Check sheet for the drawn part. Datum: minimum x, y, z corner. Units: mm. Coordinates: 2 decimals unless noted, no trailing zeros. Order: outer loops, then holes, each group sorted by start corner. A loop starts at its lowest first (then second) coordinate and runs counter-clockwise, first axis right, second up.
Q1. Cross-section at B-B, the plane x = 143. Record the boundary of the cut face in (y, z) (1 decimal), and give its area (3 significant figures).
Q2. Cross-section at A-A, the plane y = 4. Count the separate pieces of the cut face and the enclosed holes in it, and give its area (3 significant figures).
Q3. Depth check by flat-ended pin: P1, Ø3, axis at x = 66.5, y = 3, coming from the -Z side; P2, Ø3, axis at x = 112.5, y = 2.5, coming from the -Z side. Enter the tip coordinate at first touch or a pass-through.
Q4. Cross-section at C-C, the plane z = 89. Record the boundary of the cut face in (x, y) (1 decimal), and give its area (3 significant figures).
Q5. Thickness scan on line 1 (Z direction, x = 83.5, y = 4.35); line 2 (Z direction, x = 116.5, y = 4.7) (1 decimal); line 3 (X direction, y = 4.35, z = 144.5) (1 decimal). Record the ranges inside material, lowest first.
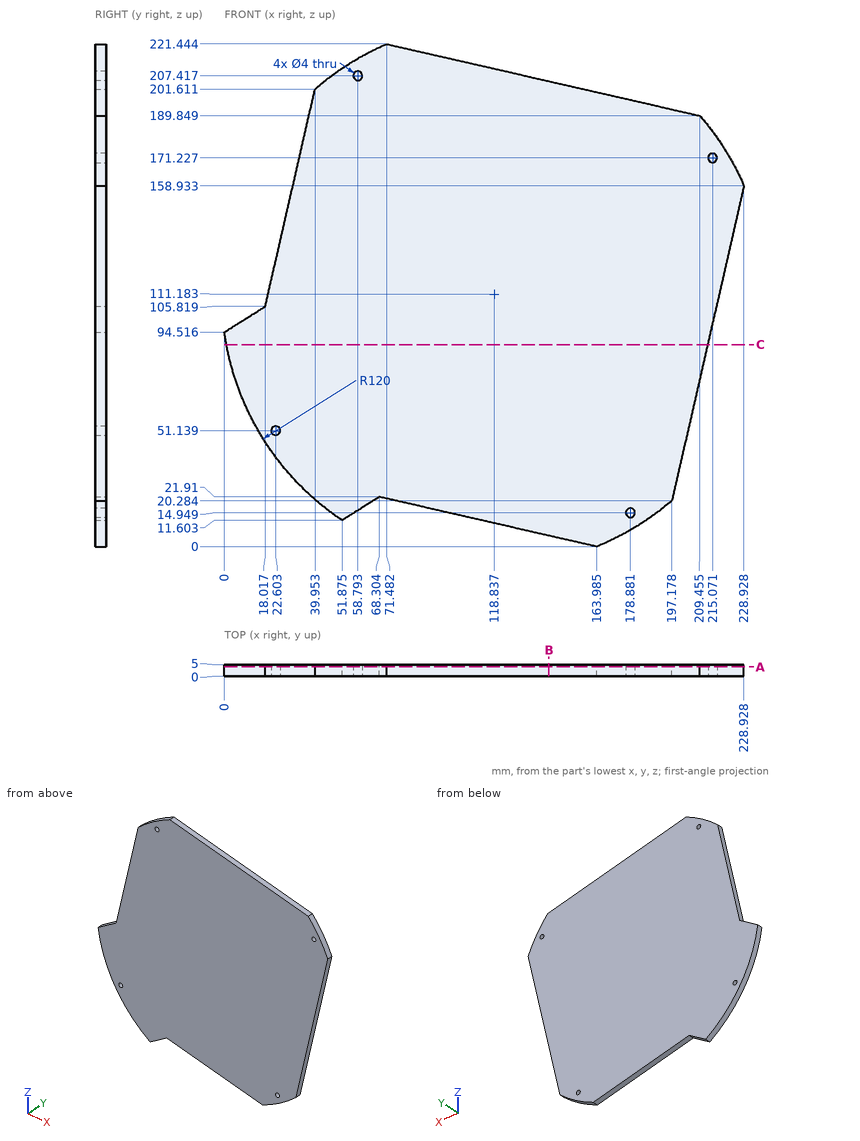
Check values:
1. outline: (0, 4.8) - (5, 4.8) - (5, 205.1) - (0, 205.1) - close
1. area: 1,000 mm2
2. separate pieces: 1
2. enclosed holes: 4
2. area: 37,100 mm2
3. P1: stops at z = 19.84
3. P2: stops at z = 11.45
4. outline: (0.9, 0) - (212.9, 0) - (212.9, 5) - (0.9, 5) - close
4. area: 1,060 mm2
5. line 1: z = 18.43 to 218.69
5. line 2: z = 10.9 to 211.1
5. line 3: x = 26.9 to 225.6
